from build123d import *

# Parameters (mm, degrees)
SKETCH1_W           = 145.9
SKETCH1_H           = 101.5
BOSS_EXTRUDE1_DEPTH = 25
CUT_EXTRUDE1_DEPTH  = 5.6
FILLET1_R           = 2
SKETCH3_R           = 1.5
CUT_EXTRUDE2_DEPTH  = 5
SKETCH4_W           = 5.2
SKETCH4_H           = 1.393306894
SKETCH4_H_2         = 0.957581617
CUT_EXTRUDE3_DEPTH  = 3
CUT_EXTRUDE4_DEPTH  = 4


with BuildPart() as part:
    # Sketch1 → Boss-Extrude1 (new body)
    with BuildSketch(Plane(origin=(0, 0, 0), x_dir=(0, 0, -1), z_dir=(1, 0, 0))):
        with Locations((9.359172662, -19.957733813)):
            Rectangle(SKETCH1_W, SKETCH1_H)
    extrude(amount=BOSS_EXTRUDE1_DEPTH)

    # Sketch2 → Cut-Extrude1 (cut)
    with BuildSketch(Plane(origin=(25, 0, 0), x_dir=(0, 0, -1), z_dir=(1, 0, 0))):
        Polygon((67.309172662, 30.792266187), (79.309172662, 18.566731656), (79.309172662, -58.929107722), (67.309172662, -70.707733813), (82.309172662, -70.707733813), (82.309172662, 30.792266187), align=None)
        Polygon((-45.590827338, 30.792266187), (-63.590827338, 15.815954922), (-63.590827338, 30.792266187), align=None)
        Polygon((-63.590827338, -62.51914727), (-55.590827338, -70.707733813), (-63.590827338, -70.707733813), align=None)
    extrude(amount=-CUT_EXTRUDE1_DEPTH, mode=Mode.SUBTRACT)

    # Fillet1
    fillet1_edges = [part.edges().sort_by_distance(p)[0] for p in [
        (9.7, 30.792266187, -82.309172662),
        (9.7, -70.707733813, -82.309172662),
        (9.7, 30.792266187, 63.590827338),
        (9.7, -70.707733813, 63.590827338),
    ]]
    fillet(fillet1_edges, radius=FILLET1_R)

    # Sketch3 → Cut-Extrude2 (cut)
    with BuildSketch(Plane.ZY):
        with Locations((-64.000619116, 27.792266187)):
            Circle(SKETCH3_R)
        with Locations((12.499380884, 27.792266187)):
            Circle(SKETCH3_R)
        with Locations((-64.000619116, -67.707733813)):
            Circle(SKETCH3_R)
        with Locations((12.499380884, -67.707733813)):
            Circle(SKETCH3_R)
    extrude(amount=-CUT_EXTRUDE2_DEPTH, mode=Mode.SUBTRACT)

    # Sketch4 → Cut-Extrude3 (cut)
    with BuildSketch(Plane(origin=(0, 0, -82.309172662), x_dir=(-1, 0, 0), z_dir=(0, 0, -1))):
        with Locations((-4.6, -65.40438726)):
            Rectangle(SKETCH4_W, SKETCH4_H)
        with Locations((-4.6, 25.271056996)):
            Rectangle(SKETCH4_W, SKETCH4_H_2)
    extrude(amount=-CUT_EXTRUDE3_DEPTH, mode=Mode.SUBTRACT)

    # Sketch5 → Cut-Extrude4 (cut)
    with BuildSketch(Plane(origin=(0, 0, -82.309172662), x_dir=(-1, 0, 0), z_dir=(0, 0, -1))):
        Polygon((0, -41.532404589), (-0.8, -41.532404589), (-0.8, -21.907733813), (-4, -21.907733813), (-4, -24.107733813), (-5.4, -24.107733813), (-5.4, -61.107733813), (-0.8, -61.107733813), (-0.8, -63.307733813), (0, -63.307733813), align=None)
    extrude(amount=-CUT_EXTRUDE4_DEPTH, mode=Mode.SUBTRACT)


solid = part.part
Read the model definition and answer for the solid it produces. Units are mm, in the model's axes. A direction names the side the tool comes from. Coordinates: 2 decimals unless noted, no trailing zeros. Loops run counter-clockwise (first coordinate to the right, second up) from the corner with the lowest first, then second, coordinate; pieces in that order, holes last. Notation, with made-up numbers: (41.5, 5.25) -> (76.5, 5.25) arc R4 cw to (76.5, 9.25) -> close; hole circle Ø1 at (-28, 74). An arc over 180 degrees is marked (long way). Answer in a Markdown table with one row per item.
Item 1: Straight lines are drawn through the part: line 1 along Z through (x, y) = (4.25, -44); line 2 along Z through (x, y) = (21, 11); line 3 along Y through (x, z) = (20, -75). For each, find the intervals that lie inside material, in ascending order. Write a range as [from, to].
Returned:
| item | result |
|---|---|
| line 1 | z = [-78.31, 63.59] |
| line 2 | z = [-79.31, 63.59] |
| line 3 | y = [-63.16, 22.96] |
Item 2: For a pull along Y with two mould halves and no side action, classify faces 1 (the flat face through (19.4, -68, 61)), 2 (the flat face through (5, 25.75, -81)), 3 (the flat face through (5, 28, 12)), 4 (the flat face through (12, -70.708, -8)) as released by +Y, released by -Y, zero draft, split by the parting line, or undercut.
Returned:
| item | result |
|---|---|
| face 1 | zero draft |
| face 2 | undercut |
| face 3 | undercut |
| face 4 | released by -Y |
Item 3: A cutting plane is placed at A-A on x = 22. Determine the outline of the cut face in (y, z), plus the area to 3 significant figures.
Returned:
| item | result |
|---|---|
| outline | (-70.71, -67.31) -> (-58.93, -79.31) -> (18.57, -79.31) -> (30.79, -67.31) -> (30.79, 45.59) -> (15.82, 63.59) -> (-62.52, 63.59) -> (-70.71, 55.59) -> close |
| area | 14,200 mm^2 |
Item 4: For faces 5 (the flat face through (19.4, 27, 58)), 6 (the flat face through (19.4, -20, -80)), 7 (the flat face through (5.4, -42, -80)), 8 (the flat face through (22.24, -64.74, -73.39)), 9 (the flat face through (22.239, -66.556, 59.647)), determine the directions among +Z, -Z, +X, -X, +Y, -Y from which every point of the face is accessible in a straight line to the end or side of a thin tool.
Returned:
| item | result |
|---|---|
| face 5 | +Z, +X, +Y |
| face 6 | -Z, +X |
| face 7 | -Z |
| face 8 | -Z, +X, -Y |
| face 9 | +Z, +X, -Y |
Item 5: Each of these flat-tipped pins is pushed along its axis until it touches: P1, Ø1.5, axis at y = -65.5, z = -80, coming from the +X side; P2, Ø1.2, axis at y = -34, z = -80, coming from the -X side; P3, Ø2.5, axis at y = 27.79, z = 12.5, coming from the -X side; P4, Ø4.5, axis at x = 1.5, y = -50.5, coming from the -Z side. Where does it stop, or does it pass through?
Returned:
| item | result |
|---|---|
| P1 | stops at x = 19.4 |
| P2 | stops at x = 0 |
| P3 | stops at x = 5 |
| P4 | stops at z = -78.31 |
